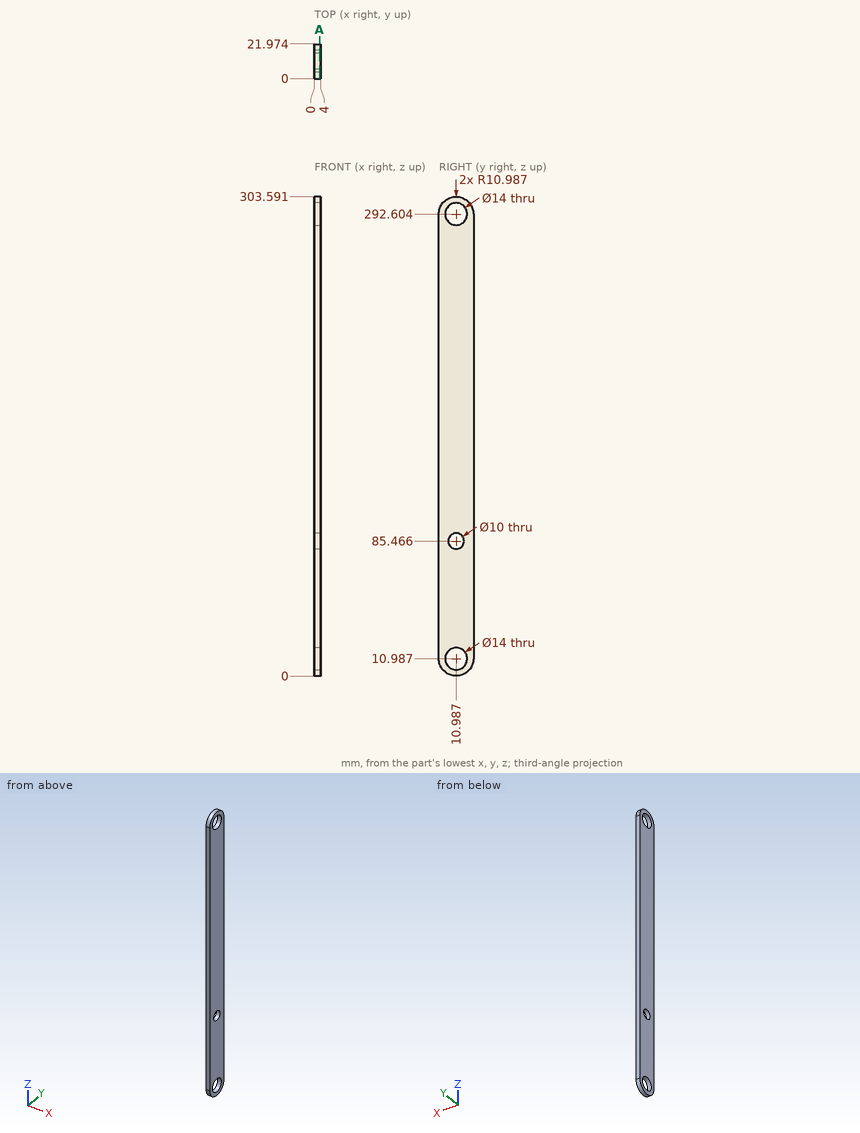
Study the drawing (mm; zero at the part's minimum x, y, z) and answer. Give positions to 0.01 mm unless a question says otherwise; leave off trailing zeros. Order: outer loops, then holes, each group sorted by start corner. A loop starts at its lowest first (then second) coordinate and runs counter-clockwise, first axis right, second up. Notation, with made-up numbers: (16, 66) - (62, 66) arc R21 ccw to (62, 104) - close; hole circle Ø2 at (30.25, 44.25). An arc over 180 degrees is marked (long way). Answer in a Markdown table with one row per item. Add a question column.
Q1. The part is cut by section A-A (x = 3.25). Determine the outline of the cut face in (y, z).
Q2. Given P1, Ø9, axis at y = 10.99, z = 85.47, coming from the -X side, flat-ended and moving along its own axis, determine where the tip first touches the part or whether it passes through.
Q3. Find the intervals of material crossed by line 1 along Z through (x, y) = (3.35, 11); line 2 along Z through (x, y) = (0.55, 7.75) (1 decimal); line 3 along Z through (x, y) = (2.1, 16.5) (1 decimal), in increasing order. Write a range as [from, to].
Determined:
| question | item | result |
|---|---|---|
| 1 | outline | (0, 10.99) arc R10.99 ccw to (21.97, 10.99) - (21.97, 292.6) arc R10.99 ccw to (0, 292.6) - close; hole circle Ø14 at (10.99, 10.99); hole circle Ø14 at (10.99, 292.6); hole circle Ø10 at (10.99, 85.47) |
| 2 | P1 | passes through |
| 3 | line 1 | z = [0, 3.99], [17.99, 80.47], [90.47, 285.6], [299.6, 303.59] |
| 3 | line 2 | z = [0.5, 4.8], [17.2, 81.7], [89.3, 286.4], [298.8, 303.1] |
| 3 | line 3 | z = [1.5, 6.7], [15.3, 288.3], [296.9, 302.1] |
